```python
from build123d import *

# Parameters (mm, degrees)
F0_R     = 2.54
F1_DEPTH = 558.8


with BuildPart() as f1:
    # F0 (on Front) → F1 (new body)
    with BuildSketch(Plane.XZ):
        with BuildLine():
            Line((241.299638, 2.54), (241.299638, 8.89))
            Line((241.299638, 8.89), (234.95, 8.89))
            ThreePointArc((234.95, 8.89), (228.6, 15.24), (222.25, 8.89))
            Line((222.25, 8.89), (215.9, 8.89))
            ThreePointArc((215.9, 8.89), (209.55, 15.24), (203.2, 8.89))
            Line((203.2, 8.89), (196.85, 8.89))
            ThreePointArc((196.85, 8.89), (190.5, 15.24), (184.15, 8.89))
            Line((184.15, 8.89), (177.8, 8.89))
            ThreePointArc((177.8, 8.89), (171.45, 15.24), (165.1, 8.89))
            Line((165.1, 8.89), (158.75, 8.89))
            ThreePointArc((158.75, 8.89), (152.4, 15.24), (146.05, 8.89))
            Line((146.05, 8.89), (139.7, 8.89))
            ThreePointArc((139.7, 8.89), (133.35, 15.24), (127, 8.89))
            Line((127, 8.89), (120.65, 8.89))
            ThreePointArc((120.65, 8.89), (114.3, 15.24), (107.95, 8.89))
            Line((107.95, 8.89), (101.6, 8.89))
            ThreePointArc((101.6, 8.89), (95.25, 15.24), (88.9, 8.89))
            Line((88.9, 8.89), (82.55, 8.89))
            ThreePointArc((82.55, 8.89), (76.2, 15.24), (69.85, 8.89))
            Line((69.85, 8.89), (63.5, 8.89))
            ThreePointArc((63.5, 8.89), (57.15, 15.24), (50.8, 8.89))
            Line((50.8, 8.89), (44.45, 8.89))
            ThreePointArc((44.45, 8.89), (38.1, 15.24), (31.75, 8.89))
            Line((31.75, 8.89), (25.4, 8.89))
            ThreePointArc((25.4, 8.89), (19.05, 15.24), (12.7, 8.89))
            Line((12.7, 8.89), (6.35, 8.89))
            ThreePointArc((6.35, 8.89), (0, 15.24), (-6.35, 8.89))
            Line((-6.35, 8.89), (-12.7, 8.89))
            ThreePointArc((-12.7, 8.89), (-19.05, 15.24), (-25.4, 8.89))
            Line((-25.4, 8.89), (-31.75, 8.89))
            ThreePointArc((-31.75, 8.89), (-38.1, 15.24), (-44.45, 8.89))
            Line((-44.45, 8.89), (-50.8, 8.89))
            ThreePointArc((-50.8, 8.89), (-57.15, 15.24), (-63.5, 8.89))
            Line((-63.5, 8.89), (-69.85, 8.89))
            ThreePointArc((-69.85, 8.89), (-76.2, 15.24), (-82.55, 8.89))
            Line((-82.55, 8.89), (-88.9, 8.89))
            ThreePointArc((-88.9, 8.89), (-95.25, 15.24), (-101.6, 8.89))
            Line((-101.6, 8.89), (-107.95, 8.89))
            ThreePointArc((-107.95, 8.89), (-114.3, 15.24), (-120.65, 8.89))
            Line((-120.65, 8.89), (-127, 8.89))
            ThreePointArc((-127, 8.89), (-133.35, 15.24), (-139.7, 8.89))
            Line((-139.7, 8.89), (-146.05, 8.89))
            ThreePointArc((-146.05, 8.89), (-152.4, 15.24), (-158.75, 8.89))
            Line((-158.75, 8.89), (-165.1, 8.89))
            ThreePointArc((-165.1, 8.89), (-171.45, 15.24), (-177.8, 8.89))
            Line((-177.8, 8.89), (-184.15, 8.89))
            ThreePointArc((-184.15, 8.89), (-190.5, 15.24), (-196.85, 8.89))
            Line((-196.85, 8.89), (-203.2, 8.89))
            ThreePointArc((-203.2, 8.89), (-209.55, 15.24), (-215.9, 8.89))
            Line((-215.9, 8.89), (-222.25, 8.89))
            ThreePointArc((-222.25, 8.89), (-228.6, 15.24), (-234.95, 8.89))
            Line((-234.95, 8.89), (-241.299638, 8.89))
            Line((-241.299638, 8.89), (-241.299638, 2.54))
            Line((-241.299638, 2.54), (-209.55, 2.54))
            Line((-209.55, 2.54), (-209.55, -3.175))
            Line((-209.55, -3.175), (-203.835, -8.89))
            Line((-203.835, -8.89), (203.835, -8.89))
            Line((203.835, -8.89), (209.55, -3.175))
            Line((209.55, -3.175), (209.55, 2.54))
            Line((209.55, 2.54), (241.299638, 2.54))
        make_face()
        with Locations((-191.163868, 0)):
            Circle(F0_R, mode=Mode.SUBTRACT)
        with Locations((-105.212435, 0)):
            Circle(F0_R, mode=Mode.SUBTRACT)
        Circle(F0_R, mode=Mode.SUBTRACT)
        with Locations((105.212435, 0)):
            Circle(F0_R, mode=Mode.SUBTRACT)
        with Locations((191.163868, 0)):
            Circle(F0_R, mode=Mode.SUBTRACT)
        with Locations((-228.6, 8.89)):
            Circle(F0_R, mode=Mode.SUBTRACT)
        with Locations((228.6, 8.89)):
            Circle(F0_R, mode=Mode.SUBTRACT)
    extrude(amount=F1_DEPTH)


solid = f1.part
```
Read the model definition and answer for the solid it produces. Units are mm, in the model's axes. A direction names the side the tool comes from. Give positions to 0.01 mm unless a question says otherwise; leave off trailing zeros. Put each result on its own line as item: value. Start each with the question number.
1. For a pull along X with two mould halves and no side action, classify faces 3 (the flat face through (-3, -275, -8.89)), 4 (the cylindrical face through (-209.41, -275.49, 15.24)) as released by +X, released by -X, zero draft, split by the parting line, or undercut.
2. Consider line 1 along X through (y, z) = (-101, -1.5); line 2 along Z through (x, y) = (69.5, -260); line 3 along X through (y, z) = (-125, -3). Determine where each line is inside the solid, lowest interval first.
3. The part is cut by section A-A, the plane y = -391. Give the number of separate pieces and of enclosed holes in the cut face, and give its area (3 significant figures).
4. Each of these flat-tipped pins is pushed along its axis until it touches: pin 1 Ø1.9 at (x, y) = (-161.5, -316.5) entering from +Z; pin 2 Ø6 at (y, z) = (-394, -3) entering from -X; pin 3 Ø7 at (x, y) = (-106.5, -289.5) entering from +Z. Where does it stop, or does it pass through?
5. Which of the six approach directions +Z, -Z, +X, -X, +Y, -Y give full straight-line access (tool end or side, diameter ignored) to faces 1 (the flat face through (225, -275, 2.54)), 2 (the cylindrical face through (-228.46, -275.49, 15.24))?
Final values:
1. face 3: zero draft
1. face 4: undercut
2. line 1: x = -209.55 to -193.21, -189.11 to -107.26, -103.16 to -2.05, 2.05 to 103.16, 107.26 to 189.11, 193.21 to 209.55
2. line 2: z = -8.89 to 8.89
2. line 3: x = -209.55 to 209.55
3. separate pieces: 1
3. enclosed holes: 7
3. area: 9,260 mm²
4. pin 1: stops at z = 8.89
4. pin 2: stops at x = -209.55
4. pin 3: stops at z = 13.56
5. face 1: -Z, +X, +Y, -Y
5. face 2: +Z, +Y, -Y
